Part model, mm, in its own coordinate system. A direction names the side the tool comes from. Give positions to 0.01 mm unless a question says otherwise; leave off trailing zeros. Write each loop counter-clockwise with the first axis right and the second up, starting at its lowest first coordinate (ties: lowest second). Pieces come first, ordered by that corner, then holes.
```python
from build123d import *

# Parameters (mm, degrees)
F0_W     = 180
F0_H     = 140
F1_DEPTH = 40
F2_W     = 130
F2_H     = 50
F2_W_2   = 140
F2_H_2   = 15
F2_W_3   = 100
F3_DEPTH = 5
F4_W     = 170
F4_H     = 130
F5_DEPTH = 25
F6_R     = 4
F7_DEPTH = 25


with BuildPart() as f1:
    # F0 (on Front) → F1 (new body)
    with BuildSketch(Plane.XZ):
        Rectangle(F0_W, F0_H)
    extrude(amount=F1_DEPTH)

    # F2 (on face) → F3 (cut)
    with BuildSketch(Plane.XZ.offset(40)):
        with Locations((0, 35)):
            Rectangle(F2_W, F2_H)
        with Locations((0, -17.5)):
            Rectangle(F2_W_2, F2_H_2)
        with Locations((0, -52.5)):
            Rectangle(F2_W_3, F2_H_2)
    extrude(amount=-F3_DEPTH, mode=Mode.SUBTRACT)

    # F4 (on face) → F5 (cut)
    with BuildSketch(Plane(origin=(0, 0, 0), x_dir=(-1, 0, 0), z_dir=(0, 1, 0))):
        Rectangle(F4_W, F4_H)
    extrude(amount=-F5_DEPTH, mode=Mode.SUBTRACT)

    # F6 (on face) → F7 (cut)
    with BuildSketch(Plane.XY.offset(70)):
        with Locations((48.596286, -20)):
            Circle(F6_R)
        with Locations((-51.403714, -20)):
            Circle(F6_R)
    extrude(amount=-F7_DEPTH, mode=Mode.SUBTRACT)


solid = f1.part
```
1) Saw through at B-B, the plane z = 50. Write the cut outline in (x, y), then the cut area to 3 significant figures.
Answers follow:
outline: (-90, -40) - (-65, -40) - (-65, -35) - (65, -35) - (65, -40) - (90, -40) - (90, 0) - (85, 0) - (85, -25) - (-85, -25) - (-85, 0) - (-90, 0) - close
area: 2,300 mm2
2) Saw through at A-A, the plane y = -20. Write the cut outline in (x, z), then the cut area to 3 significant figures.
Answers follow:
outline: (-90, -70) - (90, -70) - (90, 70) - (52.6, 70) - (52.6, 65) - (85, 65) - (85, -65) - (-85, -65) - (-85, 65) - (-55.4, 65) - (-55.4, 70) - (-90, 70) - close; (-47.4, 65) - (44.6, 65) - (44.6, 70) - (-47.4, 70) - close
area: 3,020 mm2
3) Two-plate mould, pull along Y, no slides. Class faces 1 (the face through (-1, -35, -52)), 2 (the face through (1, -25, 1)), 3 (the face through (-54.352, -17.297, 67.535)), 4 (the face through (-1, -38, 10)): +Y half, -Y half, draft (parallel to the pull), parting line (faces both ways), or undercut.
Answers follow:
face 1: -Y half
face 2: +Y half
face 3: undercut
face 4: draft
4) Wall check: L1, parallel to Z at x = 35, y = -17; L2, parallel to X at y = -5.5, z = 57.5; L3, parallel to Y at x = -36.5, z = -43.5. Give the ranges that are in metal, low to high.
Answers follow:
L1: z = -70 to -65, 65 to 70
L2: x = -90 to -85, 85 to 90
L3: y = -40 to -25
5) Pin check, flat tips, straight feed: pin 1 Ø4.5 at (x, z) = (21.5, -55) entering from -Y; pin 2 Ø7 at (x, y) = (-51.4, -20) entering from +Z; pin 3 Ø16.5 at (x, z) = (15, -16.5) entering from -Y. Stop position of each tip, or through.
Answers follow:
pin 1: stops at y = -35
pin 2: stops at z = -65
pin 3: stops at y = -40
6) Saw through at C-C, the plane x = -39. Write the cut outline in (y, z).
Answers follow:
outline: (-40, -70) - (0, -70) - (0, -65) - (-25, -65) - (-25, 65) - (0, 65) - (0, 70) - (-40, 70) - (-40, 60) - (-35, 60) - (-35, 10) - (-40, 10) - (-40, -10) - (-35, -10) - (-35, -25) - (-40, -25) - (-40, -45) - (-35, -45) - (-35, -60) - (-40, -60) - close
7) 3-axis set-ups, long thin cutter, end or side, ignore diameter. For faces 5 (the face through (-1, -38, -25)), 6 (the face through (-1, -20, -70)), 7 (the face through (1, -12, 65)): which of +Z, -Z, +X, -X, +Y, -Y reach the whole face in a straight line?
Answers follow:
face 5: -Y
face 6: -Z, +X, -X, +Y, -Y
face 7: +Y
